```python
from build123d import *

# Parameters (mm, degrees)
SKETCH1_W              = 33.02
SKETCH1_H              = 19.05
BOSS_EXTRUDE1_DEPTH    = 10.16
SKETCH2_R              = 4.7625
SKETCH2_R_2            = 2.357295936
BOSS_EXTRUDE2_DEPTH    = 10.16
SKETCH5_W              = 19.05
SKETCH5_H              = 10.16
BOSS_EXTRUDE3_DEPTH    = 5.08
SKETCH6_W              = 19.05
SKETCH6_H              = 10.16
BOSS_EXTRUDE4_DEPTH    = 5.08
SKETCH7_W              = 27.94
SKETCH7_H              = 19.05
BOSS_EXTRUDE5_DEPTH    = 128.27
SKETCH9_R              = 4.7625
BOSS_EXTRUDE6_DEPTH    = 15.24
SKETCH10_W             = 43.18
SKETCH10_H             = 138.43
CUT_EXTRUDE1_DEPTH     = 2.032
CUT_EXTRUDE2_START     = 20.955
CUT_EXTRUDE2_OUTLINE_R = 4.7625
CUT_EXTRUDE2_DEPTH     = 0.7366
SKETCH11_R             = 4.4704
BOSS_EXTRUDE7_DEPTH    = 0.7366
CUT_EXTRUDE3_START     = 16.51
CUT_EXTRUDE3_OUTLINE_R = 4.7625
CUT_EXTRUDE3_DEPTH     = 0.7366
SKETCH12_R             = 4.4704
BOSS_EXTRUDE8_DEPTH    = 0.7366


# Read off the part's stored shape, not the designer's step: Cut-Extrude2, Cut-Extrude3
with BuildPart() as part:
    # Sketch1 → Boss-Extrude1 (new body)
    with BuildSketch(Plane(origin=(0, 0, 0), x_dir=(1, 0, 0), z_dir=(0, 1, 0))):
        with Locations((-5.08, 0)):
            Rectangle(SKETCH1_W, SKETCH1_H)
    extrude(amount=BOSS_EXTRUDE1_DEPTH)

    # Sketch2 → Boss-Extrude2 (add)
    with BuildSketch(Plane(origin=(0, 10.16, 0), x_dir=(1, 0, 0), z_dir=(0, 1, 0))):
        with Locations(Location((-11.43, 0, 0), (0, 0, 270))):
            Circle(SKETCH2_R)
        with Locations(Location((1.27, 0, 0), (0, 0, 270))):
            Circle(SKETCH2_R_2)
    extrude(amount=BOSS_EXTRUDE2_DEPTH)

    # Sketch5 → Boss-Extrude3 (add)
    with BuildSketch(Plane.ZY.offset(21.59)):
        with Locations((0, 5.08)):
            Rectangle(SKETCH5_W, SKETCH5_H)
    extrude(amount=BOSS_EXTRUDE3_DEPTH)

    # Sketch6 → Boss-Extrude4 (add)
    with BuildSketch(Plane(origin=(11.43, 0, 0), x_dir=(0, 0, -1), z_dir=(1, 0, 0))):
        with Locations((0, 5.08)):
            Rectangle(SKETCH6_W, SKETCH6_H)
    extrude(amount=BOSS_EXTRUDE4_DEPTH)

    # Sketch7 → Boss-Extrude5 (add)
    with BuildSketch(Plane(origin=(0, 0, 0), x_dir=(-1, 0, 0), z_dir=(0, -1, 0))):
        with Locations((5.08, 0)):
            Rectangle(SKETCH7_W, SKETCH7_H)
    extrude(amount=BOSS_EXTRUDE5_DEPTH)

    # Sketch9 → Boss-Extrude6 (add)
    with BuildSketch(Plane.XY.offset(9.525)):
        with Locations(Location((-5.08, -123.5075, 0), (0, 0, 270))):
            Circle(SKETCH9_R)
    extrude(amount=BOSS_EXTRUDE6_DEPTH)

    # Sketch10 → Cut-Extrude1 (cut)
    with BuildSketch(Plane(origin=(0, 0, -9.525), x_dir=(-1, 0, 0), z_dir=(0, 0, -1))):
        with Locations((5.08, -59.055)):
            Rectangle(SKETCH10_W, SKETCH10_H)
    extrude(amount=-CUT_EXTRUDE1_DEPTH, mode=Mode.SUBTRACT)

    # Cut-Extrude2 outline → Cut-Extrude2 (cut)
    with BuildSketch(Plane.XY.offset(CUT_EXTRUDE2_START)):
        with Locations((-5.08, -123.5075)):
            Circle(CUT_EXTRUDE2_OUTLINE_R)
    extrude(amount=CUT_EXTRUDE2_DEPTH, mode=Mode.SUBTRACT)

    # Sketch11 → Boss-Extrude7 (add)
    with BuildSketch(Plane.XY.offset(20.955)):
        with Locations((-5.08, -123.5075)):
            Circle(SKETCH11_R)
    extrude(amount=BOSS_EXTRUDE7_DEPTH)

    # Cut-Extrude3 outline → Cut-Extrude3 (cut)
    with BuildSketch(Plane(origin=(0, 0, 0), x_dir=(1, 0, 0), z_dir=(0, 1, 0)).offset(CUT_EXTRUDE3_START)):
        with Locations((-11.43, 0)):
            Circle(CUT_EXTRUDE3_OUTLINE_R)
    extrude(amount=CUT_EXTRUDE3_DEPTH, mode=Mode.SUBTRACT)

    # Sketch12 → Boss-Extrude8 (add)
    with BuildSketch(Plane(origin=(0, 16.51, 0), x_dir=(1, 0, 0), z_dir=(0, 1, 0))):
        with Locations(Location((-11.43, 0, 0), (0, 0, 270))):
            Circle(SKETCH12_R)
    extrude(amount=BOSS_EXTRUDE8_DEPTH)


solid = part.part
```
Source: CAD feature listing. Evaluate the final solid. Frame: model axes, mm. A direction names the side the tool comes from. Round coordinates to 2 decimals unless told otherwise and drop trailing zeros. Order: outer loops, then holes, each group sorted by start corner. A loop starts at its lowest first (then second) coordinate and runs counter-clockwise, first axis right, second up. Notation, with made-up numbers: (-4, 61.5) -> (35, 61.5) arc R9 ccw to (35, 78.5) -> close; hole circle Ø10 at (10, -29.5). An arc over 180 degrees is marked (long way). Use CSV: the item, a comma, the result in double quotes.
(1) Section A-A on z = 8. Return the cut outline in (x, y).
Report:
outline,"(-26.67, 0) -> (-19.05, 0) -> (-19.05, -128.27) -> (8.89, -128.27) -> (8.89, 0) -> (16.51, 0) -> (16.51, 10.16) -> (-26.67, 10.16) -> close"
(2) Section D-D on z = 0. Return the cut outline in (x, y).
Report:
outline,"(-26.67, 0) -> (-19.05, 0) -> (-19.05, -128.27) -> (8.89, -128.27) -> (8.89, 0) -> (16.51, 0) -> (16.51, 10.16) -> (3.63, 10.16) -> (3.63, 20.32) -> (-1.09, 20.32) -> (-1.09, 10.16) -> (-6.67, 10.16) -> (-6.67, 16.51) -> (-6.96, 16.51) -> (-6.96, 17.25) -> (-6.67, 17.25) -> (-6.67, 20.32) -> (-16.19, 20.32) -> (-16.19, 17.25) -> (-15.9, 17.25) -> (-15.9, 16.51) -> (-16.19, 16.51) -> (-16.19, 10.16) -> (-26.67, 10.16) -> close"
(3) Pull-direction query (X, two-part tool) for faces 1 (the face through (2.86, 15.17, -1.74)), 2 (the face through (-4.87, -118.75, 15.16)), 3 (the face through (-11, 20.32, 0)); classes: +X half, -X half, draft (parallel to the pull), parting line (faces both ways), or undercut.
Report:
face 1,"undercut"
face 2,"parting line"
face 3,"draft"
(4) Section C-C on y = -104.5. Return the cut outline in (x, z) (3 decimals), and give its area (3 significant figures).
Report:
outline,"(-19.05, -7.493) -> (8.89, -7.493) -> (8.89, 9.525) -> (-19.05, 9.525) -> close"
area,"475 mm^2"
(5) First-contact query: pin 1 Ø5 at (x, y) = (-5.5, -12.5) entering from +Z (3 decimals); pin 2 Ø4 at (x, z) = (6.5, 7.5) entering from +Y; pin 3 Ø8.5 at (y, z) = (-63.5, -1.5) entering from -X; pin 4 Ø3 at (y, z) = (-99, 13) entering from +X. Flat tips, straight axial feed; report the tip coordinate or a pass-through.
Report:
pin 1,"z = 9.525"
pin 2,"y = 10.16"
pin 3,"x = -19.05"
pin 4,"through"
(6) Access query for faces 4 (the face through (-19.05, -63, 1)), 5 (the face through (-4.87, -118.75, 23.21)), 6 (the face through (-5.662, -119.075, 21.318)), 7 (the face through (8.89, -63, 1)), 8 (the face through (-15.655, 18.762, 2.198)). Directions: +Z, -Z, +X, -X, +Y, -Y. A direction counts if a zero-diameter tool reaches every point of the face in a straight line with its end or side. Return the directions, or none.
Report:
face 4,"+Z, -Z, -X, -Y"
face 5,"+Z"
face 6,"none"
face 7,"+Z, -Z, +X, -Y"
face 8,"+Y"
(7) Ray query, L1, parallel to X at y = -9.5, z = 0; L2, parallel to Z at x = 4, y = -13 (3 decimals); L3, parallel to Y at x = -19.5, z = 7.5. Return the intervals inside material, ascending.
Report:
L1,"-19.05 to 8.89"
L2,"-7.493 to 9.525"
L3,"0 to 10.16"
